from build123d import *

# Parameters (mm, degrees)
SKETCH1_W           = 20.5
SKETCH1_H           = 41.5
SKETCH1_R           = 7.5
BOSS_EXTRUDE2_DEPTH = 6
SKETCH1_3_W         = 37.5
SKETCH1_3_H         = 58.5
SKETCH1_3_W_2       = 20.5
SKETCH1_3_H_2       = 41.5
SKETCH1_3_R         = 2.1
BOSS_EXTRUDE3_DEPTH = 3
FILLET1_R           = 4


with BuildPart() as part:
    # Sketch1 → Boss-Extrude2 (new body)
    with BuildSketch(Plane(origin=(0, 0, 0), x_dir=(1, 0, 0), z_dir=(0, 1, 0))):
        with Locations((0, -10.05)):
            Rectangle(SKETCH1_W, SKETCH1_H)
        with Locations(Location((0, 0, 0), (0, 0, 270))):
            Circle(SKETCH1_R, mode=Mode.SUBTRACT)
    extrude(amount=BOSS_EXTRUDE2_DEPTH)

    # Sketch1_3 → Boss-Extrude3 (add)
    with BuildSketch(Plane(origin=(0, 0, 0), x_dir=(1, 0, 0), z_dir=(0, 1, 0))):
        with Locations((0, -10.05)):
            Rectangle(SKETCH1_3_W, SKETCH1_3_H)
        with Locations((0, -10.05)):
            Rectangle(SKETCH1_3_W_2, SKETCH1_3_H_2, mode=Mode.SUBTRACT)
        with Locations(Location((-5, -34.3, 0), (0, 0, 270))):
            Circle(SKETCH1_3_R, mode=Mode.SUBTRACT)
        with Locations(Location((5, -34.3, 0), (0, 0, 270))):
            Circle(SKETCH1_3_R, mode=Mode.SUBTRACT)
        with Locations(Location((-5, 14.2, 0), (0, 0, 270))):
            Circle(SKETCH1_3_R, mode=Mode.SUBTRACT)
        with Locations(Location((5, 14.2, 0), (0, 0, 270))):
            Circle(SKETCH1_3_R, mode=Mode.SUBTRACT)
    extrude(amount=BOSS_EXTRUDE3_DEPTH)

    # Fillet1
    fillet1_edges = [part.edges().sort_by_distance(p)[0] for p in [
        (18.75, 1.5, 39.3),
        (18.75, 1.5, -19.2),
        (-18.75, 1.5, -19.2),
        (-18.75, 1.5, 39.3),
        (-10.25, 4.5, -10.7),
        (10.25, 4.5, -10.7),
        (10.25, 4.5, 30.8),
        (-10.25, 4.5, 30.8),
    ]]
    fillet(fillet1_edges, radius=FILLET1_R)


solid = part.part
Model file for the job. Use its own axes, mm. A direction names the side the tool comes from. Give positions to 0.01 mm unless a question says otherwise; leave off trailing zeros. Loops run counter-clockwise (first coordinate to the right, second up) from the corner with the lowest first, then second, coordinate; pieces in that order, holes last.
1) Saw through at A-A (z = 34.3). Write the cut outline in (x, y).
2) Saw through at D-D (z = 0). Write the cut outline in (x, y), plus the area to 3 significant figures.
3) Saw through at C-C (x = 0). Write the cut outline in (y, z), plus the area to 3 significant figures.
4) Saw through at B-B (y = 3.6). Write the cut outline in (x, z), plus the area to 3 significant figures.
5) Tool access for faces 5 (the cylindrical face through (-9.047, 4.521, 29.659)), 6 (the cylindrical face through (-9.109, 4.521, -9.497)), 7 (the flat face through (0, 4, 30.8)): list every direction of +Z, -Z, +X, -X, +Y, -Y with a clear straight run to the whole face (end or side of a thin tool).
6) Wall check: line 1 (X direction, y = 1.7, z = -14.2); line 2 (Z direction, x = -4.5, y = 1.1); line 3 (Y direction, x = 14.5, z = 2). Give the ranges that are in metal, low to high.
7) Pull direction X, two halves, no side cores. Call faces 1 (the cylindrical face through (-6.278, 1.479, 32.634)), 2 (the flat face through (0, 4, -10.7)), 3 (the cylindrical face through (17.547, 1.521, 38.159)), 4 (the cylindrical face through (-17.609, 1.521, 38.097)): +X half, -X half, draft (parallel to the pull), parting line (faces both ways), or undercut.
8) Flat gauge pins, fed straight in: pin 1 Ø12 at (x, z) = (0, 0) entering from +Y; pin 2 Ø6.5 at (x, z) = (-5, -14.2) entering from +Y; pin 3 Ø1.5 at (x, y) = (-1, 5) entering from -Z; pin 4 Ø1.5 at (y, z) = (4.5, 2) entering from -X. Where does each tip first touch, or does it go through?
Answer block:
1. outline: (-18.75, 0) - (-7.1, 0) - (-7.1, 3) - (-18.75, 3) - close; (-2.9, 0) - (2.9, 0) - (2.9, 3) - (-2.9, 3) - close; (7.1, 0) - (18.75, 0) - (18.75, 3) - (7.1, 3) - close
2. outline: (-18.75, 0) - (-7.5, 0) - (-7.5, 6) - (-10.25, 6) - (-10.25, 3) - (-18.75, 3) - close; (7.5, 0) - (18.75, 0) - (18.75, 3) - (10.25, 3) - (10.25, 6) - (7.5, 6) - close
2. area: 84.0 mm2
3. outline: (0, -19.2) - (3, -19.2) - (3, -10.7) - (6, -10.7) - (6, -7.5) - (0, -7.5) - close; (0, 7.5) - (6, 7.5) - (6, 30.8) - (3, 30.8) - (3, 39.3) - (0, 39.3) - close
3. area: 210 mm2
4. outline: (-10.25, -6.7) arc R4 ccw to (-6.25, -10.7) - (6.25, -10.7) arc R4 ccw to (10.25, -6.7) - (10.25, 26.8) arc R4 ccw to (6.25, 30.8) - (-6.25, 30.8) arc R4 ccw to (-10.25, 26.8) - close; hole circle Ø15 at (0, 0)
4. area: 660 mm2
5. face 5: +Z, -X, +Y
5. face 6: -Z, -X, +Y
5. face 7: +Z, +X, -X, +Y
6. line 1: x = -18.75 to -7.1, -2.9 to 2.9, 7.1 to 18.75
6. line 2: z = -19.2 to -16.24, -12.16 to -6, 6 to 32.26, 36.34 to 39.3
6. line 3: y = 0 to 3
7. face 1: undercut
7. face 2: draft
7. face 3: +X half
7. face 4: -X half
8. pin 1: passes through
8. pin 2: stops at y = 3
8. pin 3: stops at z = -10.7
8. pin 4: stops at x = -10.25
